from build123d import *

# Parameters (mm, degrees)
F0_W           = 140
F0_H           = 84
F1_DEPTH       = 10
F2_D           = 11
F2_DEPTH       = 30
F2_CSINK_D     = 22.4
F2_CSINK_ANGLE = 90
F2_TIP         = 3.3047334047
F4_DEPTH       = 10
F5_SIZE        = 10
F6_T1_DEPTH    = 70
F6_T3_DEPTH    = 60
F7_R           = 3


# Not quite as in the source:
# - a fillet or chamfer that OpenCascade refuses, or shapes differently, is made with other operations: its cross-section is extruded or revolved along the edge and cut away or added


with BuildPart() as f1:
    # F0 (on Top) → F1 (new body)
    with BuildSketch(Plane.XY):
        with Locations((10, 2)):
            Rectangle(F0_W, F0_H)
    extrude(amount=-F1_DEPTH)

    # F2
    with Locations(Plane.XY):
        with Locations((0, 0)):
            CounterSinkHole(F2_D / 2, F2_CSINK_D / 2, depth=F2_DEPTH, counter_sink_angle=F2_CSINK_ANGLE)
            with Locations((0, 0, -(F2_DEPTH + F2_TIP / 2))):  # 118° drill point
                Cone(0, F2_D / 2, F2_TIP, mode=Mode.SUBTRACT)

    # F3 (on face) → F4 (join)
    with BuildSketch(Plane(origin=(0, 0, -10), x_dir=(1, 0, 0), z_dir=(0, 0, -1))):
        Polygon((80, 40), (-60, 40), (-60, -44), (-53, -44), (-53, 33), (80, 33), align=None)
    extrude(amount=F4_DEPTH)

    # F5
    f5_edges = [f1.edges().sort_by_distance(p)[0] for p in [
        (-56.5, 44, -20),
        (80, -36.5, -20),
    ]]
    chamfer(f5_edges, length=F5_SIZE)

    # F6: fillet of radius 10 on 4 edges, made by hand

    # F6_s2 → F6_t1 (cut)
    with BuildSketch(Plane.XY.offset(-45)):
        with BuildLine():
            ThreePointArc((-60, -30), (-57.0710678119, -37.0710678119), (-50, -40))
            Line((-50, -40), (-60, -40))
            Line((-60, -40), (-60, -30))
        make_face()
    extrude(amount=F6_T1_DEPTH, mode=Mode.SUBTRACT)

    # F6_s4 → F6_t3 (cut)
    with BuildSketch(Plane.XY.offset(-35)):
        with BuildLine():
            ThreePointArc((80, -30), (77.0710678119, -37.0710678119), (70, -40))
            Line((70, -40), (80, -40))
            Line((80, -40), (80, -30))
        make_face()
        with BuildLine():
            ThreePointArc((70, 44), (77.0710678119, 41.0710678119), (80, 34))
            Line((80, 34), (80, 44))
            Line((80, 44), (70, 44))
        make_face()
        with BuildLine():
            ThreePointArc((-50, 44), (-57.0710678119, 41.0710678119), (-60, 34))
            Line((-60, 34), (-60, 44))
            Line((-60, 44), (-50, 44))
        make_face()
    extrude(amount=F6_T3_DEPTH, mode=Mode.SUBTRACT)

    # F7
    f7_edges = [f1.edges().sort_by_distance(p)[0] for p in [
        (-53, -33, -15),
        (-53, 38.769696, -15.230304),
        (74.769696, -33, -15.230304),
        (-5.5, 0, -5.7),
    ]]
    fillet(f7_edges, radius=F7_R)


solid = f1.part
For this review, take the finished solid that the model builds, in its own axes (mm). A direction names the side the tool comes from. Give positions to 0.01 mm unless a question says otherwise; leave off trailing zeros. Loops run counter-clockwise (first coordinate to the right, second up) from the corner with the lowest first, then second, coordinate; pieces in that order, holes last.
Item 1: Take a section at B-B, the plane y = 15. State the section outline as (x, z) points, and give its area (3 significant figures).
Item 2: Take a section at A-A, the plane x = -46.5. State the section outline as (y, z) points, and give its area (3 significant figures).
Item 3: Draft analysis for pull direction X (two halves, no side actions). For faces 1 (the cylindrical face through (-57.15, -36.99, -10.14)), 2 (the cylindrical face through (1.19, -5.37, -8.49)), 3 (the flat face through (12, 5, -10)), 4 (the conical face through (-3.051, -5.867, -4.587)), state which applies: +X half, -X half, draft (parallel to the pull), parting line (faces both ways), or undercut.
Item 4: Tool access review of faces 5 (the flat face through (12, -33, -15)), 6 (the flat face through (-58, 37, -17)): name each direction out of +Z, -Z, +X, -X, +Y, -Y from which nothing blocks a thin tool from reaching the whole face with its end or side.
Item 5: Insertion check: pin 1 (11 mm diameter, centred on y = 7, z = -16, fed in from +X); pin 2 (5 mm diameter, centred on x = 24.5, y = -5, fed in from -Z); pin 3 (3 mm diameter, centred on x = -14, z = -14.5, fed in from +Y). Each pin has a flat end and moves straight along its axis. Give the tip position at first contact, or say it passes through.
Item 6: For line 1 along Y through (x, z) = (0, -9); line 2 along X through (y, z) = (0, -8.9); line 3 along Z through (x, y) = (65, 11), list the stretches that pass through material, from the lowest coordinate up.
Calculated:
1. outline: (-60, -20) - (-53, -20) - (-53, -10) - (80, -10) - (80, 0) - (-60, 0) - close
1. area: 1,470 mm2
2. outline: (-40, -20) - (-33, -20) - (-33, -10) - (44, -10) - (44, 0) - (-40, 0) - close
2. area: 910 mm2
3. face 1: -X half
3. face 2: undercut
3. face 3: draft
3. face 4: undercut
4. face 5: -Z, +X, +Y
4. face 6: -Z, +X, -X, +Y
5. pin 1: stops at x = -53
5. pin 2: stops at z = -10
5. pin 3: stops at y = -33
6. line 1: y = -40 to -5.5, 5.5 to 44
6. line 2: x = -60 to -5.5, 5.5 to 80
6. line 3: z = -10 to 0
